Autodesk Inventor part; units mm, degrees
ref_plane "YZ Plane" through (0, 0, 0) normal (1, 0, 0) x (0, 1, 0)
ref_plane "XZ Plane" through (0, 0, 0) normal (0, 1, 0) x (-1, 0, 0)
ref_plane "XY Plane" through (0, 0, 0) normal (0, 0, 1) x (1, 0, 0)
sketch "Sketch3" plane through (0, 0, 0) normal (0, 1, 0) x (-1, 0, 0)
  circle A0 centre (0, 0) radius 7.5
  line L0 (0, 0) -> (15, 0)
  line L1 (0, 0) -> (15, 0) construction
  line L2 (15, 0) -> (15, -3.75)
  line L3 (15, -3.75) -> (-15, -3.75)
  line L4 (-15, -3.75) -> (-15, 3.75)
  line L5 (-15, 3.75) -> (15, 3.75)
  line L6 (15, 3.75) -> (15, -3.75)
  dimension "d27" = 15
  dimension "d28" = 15
  dimension "d29" = 0
  dimension "d30" = 3.75
  dimension "d31" = 90
  dimension "d32" = 30
  dimension "d33" = 7.5
extrude "Extrusion3" add sketch "Sketch3" along normal blind 10
sketch "Sketch5" plane through (0, 0, 0) normal (0, -1, 0) x (1, 0, 0)
  circle A0 centre (0, 0) radius 5
  line L0 (0, 2.5) -> (0, -2.5)
  dimension "d39" = 10
extrude "Extrusion5" add sketch "Sketch5" along normal blind 45
sketch "Sketch6" plane through (0, 10, 0) normal (0, 1, 0) x (1, 0, 0)
  circle A0 centre (0, 0) radius 2.5
  dimension "d44" = 5
extrude "Extrusion6" cut sketch "Sketch6" against normal blind 60
sketch "Sketch7" plane through (0, 10, 0) normal (0, 1, 0) x (1, 0, 0)
  line L0 (0, 0) -> (2.5, 0)
  line L1 (2.5, 0) -> (1.5, 0)
  line L2 (2.5, 0) -> (3.5, 0) construction
  line L3 (1.5, 0) -> (1.5, -3.2812)
  line L4 (1.5, -3.2812) -> (1.5, 3.3122)
  arc A0 (1.5, -2) -> (1.5, 2) centre (0, 0) ccw
  line L5 (1.5, -2) -> (1.5, 2)
  dimension "d50" = 1
  dimension "d51" = 180
extrude "Extrusion9" add sketch "Sketch7" against normal blind 55
sketch "Sketch8" plane through (15, 0, 3.75) normal (1, 0, 0) x (0, 0, -1)
  line L0 (0, 0) -> (0, 10)
  line L1 (0, 0) -> (7.5, 0)
  circle A0 centre (3.75, 4.7055) radius 2.5
  point P0 (3.75, 0)
  dimension "d58" = 5
extrude "Extrusion10" cut sketch "Sketch8" against normal blind 15
thread "Thread2"
properties part number "Stepper_Key"
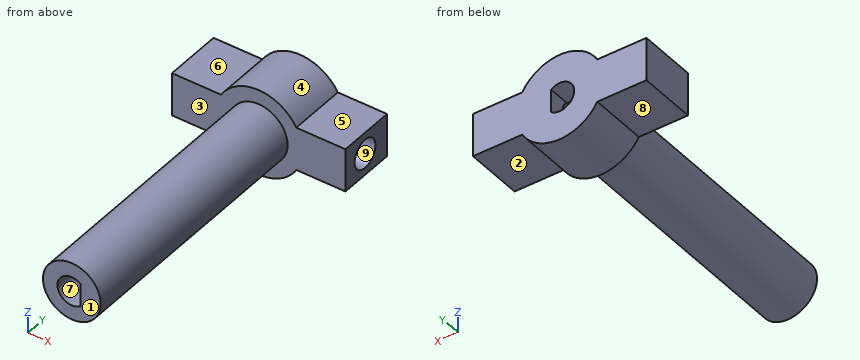
Can you work these out from the model? Positions are in its coordinate system, mm. Face numbers are marked on the shaded views. A direction names the side the tool comes from. Coordinates: 2 decimals unless noted, no trailing zeros. Loops run counter-clockwise (first coordinate to the right, second up) from the corner with the lowest first, then second, coordinate; pieces in that order, holes last.
1) Imagine slicing it at C-C on y = -22.5. List the corners of the cut face in (x, z) for me, plus the area to 3 significant figures.
2) Imagine slicing it at B-B on x = 3.5. List the corners of the cut face in (y, z) for me.
3) I need wall thicknesses on probe 1 along Z at (x, y) = (0, -26.5); probe 2 along Y at (x, z) = (13.25, 3.25); probe 3 along X at (y, z) = (-19, 0.75). Which ranges of each line are inside material? Lowest first, please.
4) Which directions (+Z, -Z, +X, -X, +Y, -Y) give clear straight access to the entire face, cutting with the end or side of a thin tool? Please do the marked faces 1, 2, 3, 4 and 5.
5) Thinking about a two-plate mould opening in Z: for the marked faces 6, 7, 8 and 9, which applies, pulls with the +Z half, pulls with the -Z half, needs draft (parallel to the pull), parting line crosses it, or undercut?
6) For pin 1 (1 mm diameter, centred on x = 3.5, y = -22.5, fed in from +Z); pin 2 (8 mm diameter, centred on x = -3.5, y = -14.5, fed in from -Z); pin 3 (6 mm diameter, centred on y = -25.5, z = 2.5, fed in from +X), each with a flat end and sliding along its axis, tell me the tip position at first contact or that it passes through.
7) Imagine slicing it at D-D on x = -11.75. List the corners of the cut face in (y, z) for me.
8) Imagine slicing it at A-A on z = 0. List the corners of the cut face in (x, y) for me, plus the area to 4 significant figures.
Completed:
1. outline: circle Ø10 at (0, 0); hole (1.5, -2) - (1.5, 2) arc R2.5 ccw (long way) to start
1. area: 61.7 mm2
2. outline: (-45, -3.57) - (0, -3.57) - (0, -6.63) - (10, -6.63) - (10, 6.63) - (0, 6.63) - (0, 3.57) - (-45, 3.57) - close; hole circle Ø5 at (4.71, 0)
3. probe 1: z = -5 to -2.5, 2.5 to 5
3. probe 2: y = 0 to 10
3. probe 3: x = -4.94 to -2.38, 1.5 to 4.94
4. face 1: +Z, -Z, +X, -X, -Y
4. face 2: -Z, +X, +Y, -Y
4. face 3: -Y
4. face 4: +Z, +Y, -Y
4. face 5: +Z, +X, +Y, -Y
5. face 6: pulls with the +Z half
5. face 7: undercut
5. face 8: pulls with the -Z half
5. face 9: undercut
6. pin 1: stops at z = 4
6. pin 2: stops at z = -5
6. pin 3: stops at x = 5
7. outline: (0, -3.75) - (10, -3.75) - (10, 3.75) - (0, 3.75) - close
8. outline: (-15, 0) - (-5, 0) - (-5, -45) - (-2.5, -45) - (-2.5, 10) - (-15, 10) - close; (1.5, -45) - (5, -45) - (5, 0) - (15, 0) - (15, 2.21) - (1.5, 2.21) - close; (1.5, 7.21) - (15, 7.21) - (15, 10) - (1.5, 10) - close
8. area: 462.5 mm2
